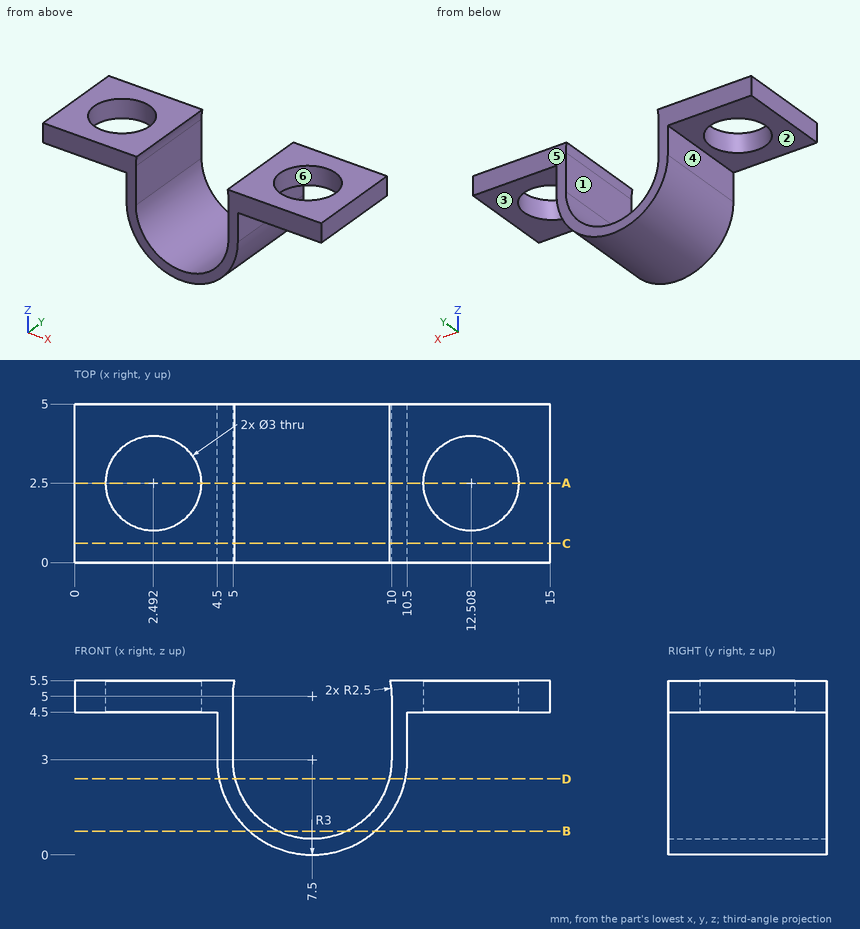
Input: dimensioned drawing with shaded views. Units: mm. Origin: part minimum x, y, z. A direction names the side the tool comes from. Round coordinates to 2 decimals unless told otherwise and drop trailing zeros. Order: outer loops, then holes, each group sorted by start corner. A loop starts at its lowest first (then second) coordinate and runs counter-clockwise, first axis right, second up. Notation, with made-up numbers: (-7, 25.5) - (3, 25.5) arc R29 ccw to (3, 56.5) - close; hole circle Ø6 at (-3.75, -19). An arc over 180 degrees is marked (long way). Answer as a JSON object with one key per item and string values. Group by question number.
(1) Cut plane B-B (z = 0.75). Return loops of the section in (x, y) (1 decimal).
(2) Reachability of the marked faces 1, 2 and 3 from +Z, -Z, +X, -X, +Y, -Y: full face, straight path, thin tool, end or side. Return the list, or none.
(3) Cut plane D-D (z = 2.4). Return loops of the section in (x, y).
(4) Cut plane C-C (y = 0.6). Return loops of the section in (x, z).
(5) Cut plane A-A (y = 2.5). Return loops of the section in (x, z).
(6) Pin query (flat end, axial travel): P1, Ø0.8, axis at y = 2.5, z = 3.5, coming from the -X side; P2, Ø1.8, axis at x = 12.51, y = 2.5, coming from the -Z side; P3, Ø0.6, axis at y = 2, z = 4, coming from the +X side; P4, Ø2, axis at x = 12, y = 3.5, coming from the -Z side. Return the tip coordinate at first contact, or that it passes through.
(7) Draft query along Y for the marked faces 4, 5 and 6. Return one class per face: released by +Y, released by -Y, zero draft, split by the parting line, or undercut.
(8) Material intervals for probe 1 along X at (y, z) = (4.2, 2); probe 2 along X at (y, z) = (1.7, 4.75); probe 3 along X at (y, z) = (2.9, 1.25) (1 decimal), sorted ascending. Write a range as from..to.
Here are the results:
{
 "1": {"outline": "(5.5, 0) - (6.4, 0) - (6.4, 5) - (5.5, 5) - close; (8.6, 0) - (9.5, 0) - (9.5, 5) - (8.6, 5) - close"},
 "2": {"face 1": "+Y, -Y", "face 2": "-Z, -X, +Y, -Y", "face 3": "-Z, +X, +Y, -Y"},
 "3": {"outline": "(4.56, 0) - (5.07, 0) - (5.07, 5) - (4.56, 5) - close; (9.93, 0) - (10.44, 0) - (10.44, 5) - (9.93, 5) - close"},
 "4": {"outline": "(0, 4.5) - (4.5, 4.5) - (4.5, 3) arc R3 ccw to (10.5, 3) - (10.5, 4.5) - (15, 4.5) - (15, 5.5) - (9.95, 5.5) arc R2.5 cw to (10, 5) - (10, 3) arc R2.5 cw to (5, 3) - (5, 5) arc R2.5 cw to (5.05, 5.5) - (0, 5.5) - close"},
 "5": {"outline": "(0, 4.5) - (0.99, 4.5) - (0.99, 5.5) - (0, 5.5) - close; (3.99, 4.5) - (4.5, 4.5) - (4.5, 3) arc R3 ccw to (10.5, 3) - (10.5, 4.5) - (11.01, 4.5) - (11.01, 5.5) - (9.95, 5.5) arc R2.5 cw to (10, 5) - (10, 3) arc R2.5 cw to (5, 3) - (5, 5) arc R2.5 cw to (5.05, 5.5) - (3.99, 5.5) - close; (14.01, 4.5) - (15, 4.5) - (15, 5.5) - (14.01, 5.5) - close"},
 "6": {"P1": "stops at x = 4.5", "P2": "passes through", "P3": "stops at x = 10.5", "P4": "stops at z = 4.5"},
 "7": {"face 4": "zero draft", "face 5": "released by +Y", "face 6": "undercut"},
 "8": {"probe 1": "x = 4.67..5.21, 9.79..10.33", "probe 2": "x = 0..1.22, 3.76..5, 10..11.24, 13.78..15", "probe 3": "x = 5.1..5.7, 9.3..9.9"}
}
